Design review of the part built by this model. Coordinates are the model's own, in mm. Give positions to 0.01 mm unless a question says otherwise; leave off trailing zeros. Write each loop counter-clockwise with the first axis right and the second up, starting at its lowest first coordinate (ties: lowest second). Pieces come first, ordered by that corner, then holes. Notation, with made-up numbers: (40.5, 89) -> (91.5, 89) arc R28 ccw to (91.5, 122) -> close; hole circle Ø11 at (63.25, 23). An arc over 180 degrees is marked (long way). Answer as a JSON object with one key per item and string values.
```python
from build123d import *

# Parameters (mm, degrees)
EXTRUDE_1_DEPTH = 5


with BuildPart() as part:
    # 草图1 → 凸台-拉伸1 (new body)
    with BuildSketch(Plane.XY):
        with BuildLine():
            ThreePointArc((0, 7), (4.949747468, 4.949747468), (7, 0))
            Line((7, 0), (48.26, 0))
            ThreePointArc((48.26, 0), (50.310252532, 4.949747468), (55.26, 7))
            Line((55.26, 7), (0, 7))
        make_face()
        with BuildLine():
            ThreePointArc((55.26, 7), (50.310252532, 4.949747468), (48.26, 0))
            Line((48.26, 0), (51.21, 0))
            ThreePointArc((51.21, 0), (55.26, 4.05), (59.31, 0))
            Line((59.31, 0), (62.26, 0))
            ThreePointArc((62.26, 0), (60.209747468, 4.949747468), (55.26, 7))
        make_face()
        with BuildLine():
            Line((51.21, 0), (48.26, 0))
            ThreePointArc((48.26, 0), (50.310252532, -4.949747468), (55.26, -7))
            ThreePointArc((55.26, -7), (60.209747468, -4.949747468), (62.26, 0))
            Line((62.26, 0), (59.31, 0))
            ThreePointArc((59.31, 0), (55.26, -4.05), (51.21, 0))
        make_face()
        with BuildLine():
            Line((48.26, 0), (7, 0))
            ThreePointArc((7, 0), (4.949747468, -4.949747468), (0, -7))
            Line((0, -7), (55.26, -7))
            ThreePointArc((55.26, -7), (50.310252532, -4.949747468), (48.26, 0))
        make_face()
        with BuildLine():
            ThreePointArc((-4.05, 0), (0, 4.05), (4.05, 0))
            Line((4.05, 0), (7, 0))
            ThreePointArc((7, 0), (4.949747468, 4.949747468), (0, 7))
            ThreePointArc((0, 7), (-4.949747468, 4.949747468), (-7, 0))
            Line((-7, 0), (-4.05, 0))
        make_face()
        with BuildLine():
            Line((7, 0), (4.05, 0))
            ThreePointArc((4.05, 0), (0, -4.05), (-4.05, 0))
            Line((-4.05, 0), (-7, 0))
            ThreePointArc((-7, 0), (-4.949747468, -4.949747468), (0, -7))
            ThreePointArc((0, -7), (4.949747468, -4.949747468), (7, 0))
        make_face()
    extrude(amount=EXTRUDE_1_DEPTH)


solid = part.part
```
(1) The part is to be moulded in two halves that separate along Y. For faces 1 (the flat face through (27, 0, 0)), 2 (the cylindrical face through (59, 1.55, 2.46)), 3 (the flat face through (27, -7, 2)), 4 (the cylindrical face through (-0.527, -4.016, 2.465)), say which applies: +Y half, -Y half, draft (parallel to the pull), parting line (faces both ways), or undercut.
Here are the results:
{"face 1": "draft", "face 2": "undercut", "face 3": "-Y half", "face 4": "undercut"}
(2) We need section B-B, the plane x = 57. State the section outline as (y, z) points.
Here are the results:
{"outline": "(-6.78, 0) -> (-3.66, 0) -> (-3.66, 5) -> (-6.78, 5) -> close; (3.66, 0) -> (6.78, 0) -> (6.78, 5) -> (3.66, 5) -> close"}
(3) For line 1 along X through (y, z) = (0.25, 4.25); line 2 along X through (y, z) = (-2.75, 2.5); line 3 along Y through (x, z) = (55.26, 3.7), list the stretches that pass through material, from the lowest coordinate up.
Here are the results:
{"line 1": "x = -7 to -4.04, 4.04 to 51.22, 59.3 to 62.26", "line 2": "x = -6.44 to -2.97, 2.97 to 52.29, 58.23 to 61.7", "line 3": "y = -7 to -4.05, 4.05 to 7"}
(4) Clearance check with flat-ended pins moving along their axes: pin 1 (6.5 mm diameter, centred on x = 55.26, y = 0, fed in from +Z); pin 2 (3 mm diameter, centred on y = 3.5, z = 4, fed in from +X). State where each tip first meets the part, or that it passes through.
Here are the results:
{"pin 1": "passes through", "pin 2": "stops at x = 61.97"}
(5) We need section A-A, the plane z = 3.95. State the section outline as (x, y) points, then the cut area to 3 significant figures.
Here are the results:
{"outline": "(0, -7) -> (55.26, -7) arc R7 ccw to (55.26, 7) -> (0, 7) arc R7 ccw to start; hole circle Ø8.1 at (0, 0); hole circle Ø8.1 at (55.26, 0)", "area": "825 mm²"}
(6) We need section D-D, the plane y = -6. State the section outline as (x, z) points.
Here are the results:
{"outline": "(-3.61, 0) -> (58.87, 0) -> (58.87, 5) -> (-3.61, 5) -> close"}
(7) We need section C-C, the plane y = 5.75. State the section outline as (x, z) points.
Here are the results:
{"outline": "(-3.99, 0) -> (59.25, 0) -> (59.25, 5) -> (-3.99, 5) -> close"}
